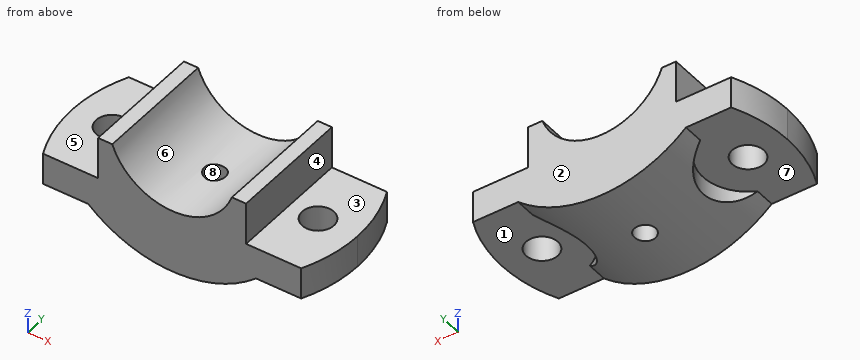
```python
from build123d import *

# Parameters (mm, degrees)
BOSS_EXTRUDE1_DEPTH = 46
SKETCH2_R           = 6
CUT_EXTRUDE1_DEPTH  = 77.26270386
SKETCH3_R           = 4
CUT_EXTRUDE2_DEPTH  = 24
CUT_EXTRUDE4_START  = 48
SKETCH2_5_R         = 6
CUT_EXTRUDE4_DEPTH  = 48


with BuildPart() as part:
    # Sketch1 → Boss-Extrude1 (new body)
    with BuildSketch(Plane(origin=(0, 0, 0), x_dir=(1, 0, 0), z_dir=(0, 1, 0))):
        with BuildLine():
            Line((-54, 0), (-28, 0))
            Line((-28, 0), (-28, -16))
            Line((-28, -16), (-22.627416998, -16))
            ThreePointArc((-22.627416998, -16), (0, 0), (22.627416998, -16))
            Line((22.627416998, -16), (28, -16))
            Line((28, -16), (28, 0))
            Line((28, 0), (54, 0))
            Line((54, 0), (54, 12))
            Line((54, 12), (31.749015733, 12))
            ThreePointArc((31.749015733, 12), (0, 24), (-31.749015733, 12))
            Line((-31.749015733, 12), (-54, 12))
            Line((-54, 12), (-54, 0))
        make_face()
    extrude(amount=BOSS_EXTRUDE1_DEPTH)

    # Sketch2 → Cut-Extrude1 (cut, through all)
    with BuildSketch(Plane(origin=(0, 0, -12), x_dir=(-1, 0, 0), z_dir=(0, 0, -1))):
        with BuildLine():
            Line((-48.856934001, 46), (-54, 46))
            Line((-54, 46), (-54, 23))
            ThreePointArc((-54, 23), (-52.698550436, 34.784005345), (-48.856934001, 46))
        make_face()
        with BuildLine():
            ThreePointArc((-48.856934001, 0), (-52.698550436, 11.215994655), (-54, 23))
            Line((-54, 23), (-54, 0))
            Line((-54, 0), (-48.856934001, 0))
        make_face()
        with Locations((-39, 23)):
            Circle(SKETCH2_R)
        with Locations((39, 23)):
            Circle(SKETCH2_R)
        with BuildLine():
            Line((54, 23), (54, 46))
            Line((54, 46), (48.856934001, 46))
            ThreePointArc((48.856934001, 46), (52.698550436, 34.784005345), (54, 23))
        make_face()
        with BuildLine():
            Line((54, 0), (54, 23))
            ThreePointArc((54, 23), (52.698550436, 11.215994655), (48.856934001, 0))
            Line((48.856934001, 0), (54, 0))
        make_face()
    extrude(amount=-CUT_EXTRUDE1_DEPTH, mode=Mode.SUBTRACT)

    # Sketch3 → Cut-Extrude2 (cut, symmetric)
    with BuildSketch(Plane(origin=(0, 0, -12), x_dir=(-1, 0, 0), z_dir=(0, 0, -1))):
        with Locations((0, 23)):
            Circle(SKETCH3_R)
    extrude(amount=CUT_EXTRUDE2_DEPTH, both=True, mode=Mode.SUBTRACT)

    # Sketch2_5 → Cut-Extrude4 (cut)
    # profile 1 of 3: a face of its own
    with BuildSketch(Plane(origin=(0, 0, -12), x_dir=(-1, 0, 0), z_dir=(0, 0, -1)).offset(CUT_EXTRUDE4_START)):
        with BuildLine():
            Line((-39, 0), (-39, 6))
            ThreePointArc((-39, 6), (-22, 23), (-39, 40))
            Line((-39, 40), (-39, 46))
            Line((-39, 46), (-48.856934001, 46))
            ThreePointArc((-48.856934001, 46), (-54, 23), (-48.856934001, 0))
            Line((-48.856934001, 0), (-39, 0))
        make_face()
        with Locations((-39, 23)):
            Circle(SKETCH2_5_R, mode=Mode.SUBTRACT)
    # profile 2 of 3: a face of its own
    with BuildSketch(Plane(origin=(0, 0, -12), x_dir=(-1, 0, 0), z_dir=(0, 0, -1)).offset(CUT_EXTRUDE4_START)):
        with BuildLine():
            ThreePointArc((48.856934001, 0), (52.698550436, 11.215994655), (54, 23))
            ThreePointArc((54, 23), (52.698550436, 34.784005345), (48.856934001, 46))
            Line((48.856934001, 46), (39, 46))
            Line((39, 46), (39, 40))
            ThreePointArc((39, 40), (35.284695392, 39.589047943), (31.749015733, 38.376060196))
            Line((31.749015733, 38.376060196), (31.749015733, 7.623939804))
            ThreePointArc((31.749015733, 7.623939804), (35.284695392, 6.410952057), (39, 6))
            Line((39, 6), (39, 0))
            Line((39, 0), (48.856934001, 0))
        make_face()
        with Locations((39, 23)):
            Circle(SKETCH2_5_R, mode=Mode.SUBTRACT)
    # profile 3 of 3: a face of its own
    with BuildSketch(Plane(origin=(0, 0, -12), x_dir=(-1, 0, 0), z_dir=(0, 0, -1)).offset(CUT_EXTRUDE4_START)):
        with BuildLine():
            Line((31.749015733, 7.623939804), (31.749015733, 38.376060196))
            ThreePointArc((31.749015733, 38.376060196), (22, 23), (31.749015733, 7.623939804))
        make_face()
    extrude(amount=-CUT_EXTRUDE4_DEPTH, mode=Mode.SUBTRACT)


solid = part.part
```
Verification items for the finished model (mm, model axes). Face numbers are marked on the shaded views. A direction names the side the tool comes from. Give positions to 0.01 mm unless a question says otherwise; leave off trailing zeros. Write each loop counter-clockwise with the first axis right and the second up, starting at its lowest first coordinate (ties: lowest second). Pieces come first, ordered by that corner, then holes. Notation, with made-up numbers: (-34, 74.25) - (-18, 74.25) arc R27 ccw to (-18, 90.25) - close; hole circle Ø6 at (-1.75, 52). An arc over 180 degrees is marked (long way). Put each result on its own line as item: value.
Q1. Section check A-A on z = -5.5. Record the cut outline in (x, y), and give its area (3 significant figures).
Result:
outline: (-48.86, 0) - (48.86, 0) arc R54 ccw to (48.86, 46) - (-48.86, 46) arc R54 ccw to start; hole circle Ø12 at (-39, 23); hole circle Ø8 at (0, 23); hole circle Ø12 at (39, 23)
area: 4,540 mm2
Q2. Mould release check, pull along Y, two halves, no side actions. Record for the marked faces 1, 2 and 3: released by +Y, released by -Y, zero draft, split by the parting line, or undercut.
Result:
face 1: undercut
face 2: released by +Y
face 3: zero draft
Q3. Section check C-C on z = 8. Record the cut outline in (x, y).
Result:
outline: (-28, 0) - (-17.89, 0) - (-17.89, 46) - (-28, 46) - close; (17.89, 0) - (28, 0) - (28, 46) - (17.89, 46) - close
Q4. Scan lines: probe 1 along Y at (x, z) = (-39, -2.25); probe 2 along Y at (x, z) = (0, -5.25); probe 3 along Z at (x, y) = (47, 42). Record each from-to range of solid material in increasing order. Write a range as from..to.
Result:
probe 1: 0..17, 29..46
probe 2: 0..19, 27..46
probe 3: -12..0
Q5. Section check B-B on x = 0. Record the cut outline in (y, z), and give its area (3 significant figures).
Result:
outline: (0, -24) - (19, -24) - (19, 0) - (0, 0) - close; (27, -24) - (46, -24) - (46, 0) - (27, 0) - close
area: 912 mm2
Q6. Set-up check for the marked faces 4, 5, 6, 7 and 8: record each of +Z, -Z, +X, -X, +Y, -Y from which the full face is reachable in a straight line by a thin tool's end or side.
Result:
face 4: +Z, +X, +Y, -Y
face 5: +Z, -X, +Y, -Y
face 6: +Z, +Y, -Y
face 7: -Z, -X
face 8: +Z, -Z
Q7. Depth check by flat-ended pin: P1, Ø7, axis at x = 39, y = 23, coming from the -Z side; P2, Ø6, axis at x = 42, z = -12.5, coming from the +Y side; P3, Ø8, axis at x = 38, y = 32.5, coming from the +Z side; P4, Ø4, axis at x = -25, y = 27, coming from the -Z side. Enter the tip coordinate at first touch or a pass-through.
Result:
P1: through
P2: y = 46
P3: z = 0
P4: z = -12
Q8. Section check D-D on x = 26. Record the cut outline in (y, z).
Result:
outline: (0, -16.35) - (12.05, -16.35) - (12.05, -12) - (33.95, -12) - (33.95, -16.35) - (46, -16.35) - (46, 16) - (0, 16) - close
